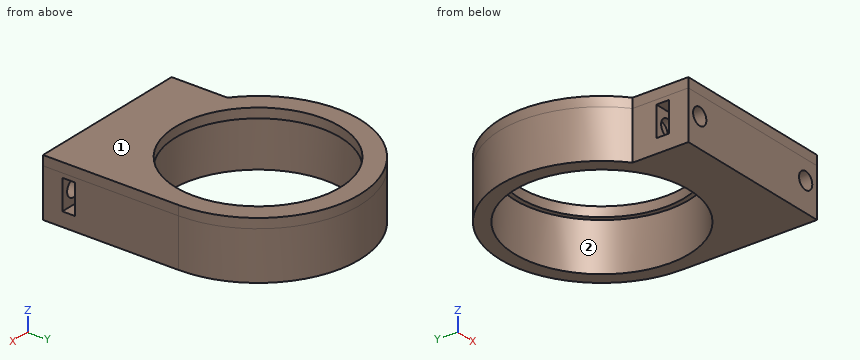
```python
from build123d import *
from build123d.topology import SkipClean

# Parameters (mm, degrees)
CROQUIS1_R              = 18
SALIENTE_EXTRUIR1_DEPTH = 10
CROQUIS2_R              = 17
SALIENTE_EXTRUIR2_DEPTH = 2
CROQUIS7_R              = 1.75
CORTAR_EXTRUIR3_DEPTH   = 8
CORTAR_EXTRUIR4_DEPTH   = 2.6


with BuildPart() as part:
    # Croquis1 → Saliente-Extruir1 (new body)
    with BuildSketch(Plane.XY):
        with BuildLine():
            Line((-13, -28), (21, -28))
            Line((21, -28), (21, 0))
            ThreePointArc((21, 0), (-9.16515139, 18.894443628), (-13, -16.492422502))
            Line((-13, -16.492422502), (-13, -28))
        make_face()
        Circle(CROQUIS1_R, mode=Mode.SUBTRACT)
    extrude(amount=SALIENTE_EXTRUIR1_DEPTH)

    # Croquis2 → Saliente-Extruir2 (add)
    with SkipClean():  # the faces are left unmerged after this step: merging them gives an invalid solid
        with BuildSketch(Plane.XY.offset(10)):
            with BuildLine():
                Line((21, 0), (21, -28))
                Line((21, -28), (-13, -28))
                Line((-13, -28), (-13, -16.492422502))
                ThreePointArc((-13, -16.492422502), (-9.16515139, 18.894443628), (21, 0))
            make_face()
            Circle(CROQUIS2_R, mode=Mode.SUBTRACT)
        extrude(amount=SALIENTE_EXTRUIR2_DEPTH)

    # Croquis7 → Cortar-Extruir3 (cut)
    with SkipClean():  # the faces are left unmerged after this step: merging them gives an invalid solid
        with BuildSketch(Plane.XZ.offset(28)):
            with Locations((-10, 6)):
                Circle(CROQUIS7_R)
            with Locations((18, 6)):
                Circle(CROQUIS7_R)
        extrude(amount=-CORTAR_EXTRUIR3_DEPTH, mode=Mode.SUBTRACT)

    # Croquis8 → Cortar-Extruir4 (cut)
    with SkipClean():  # the faces are left unmerged after this step: merging them gives an invalid solid
        with BuildSketch(Plane(origin=(0, -24, 0), x_dir=(-1, 0, 0), z_dir=(0, -1, 0))):
            with BuildLine():
                Line((-18, -2.9), (-21, -2.9))
                Line((-21, -2.9), (-21, -9.1))
                Line((-21, -9.1), (-18, -9.1))
                ThreePointArc((-18, -9.1), (-14.9, -6), (-18, -2.9))
            make_face()
            with BuildLine():
                Line((10, -2.9), (13, -2.9))
                Line((13, -2.9), (13, -9.1))
                Line((13, -9.1), (10, -9.1))
                ThreePointArc((10, -9.1), (6.9, -6), (10, -2.9))
            make_face()
        extrude(amount=-CORTAR_EXTRUIR4_DEPTH, mode=Mode.SUBTRACT)


solid = part.part
```
Geometry: final body of the model. Coordinates: model frame, mm. Face numbers are marked on the shaded views. A direction names the side the tool comes from. Coordinates: 2 decimals unless noted, no trailing zeros. Order: outer loops, then holes, each group sorted by start corner. A loop starts at its lowest first (then second) coordinate and runs counter-clockwise, first axis right, second up. Notation, with made-up numbers: M 83.25,5.25 L 107.25,5.25 A24 cw 107.25,33.25 Z; hole C -28,-24.5 d11. An arc over 180 degrees is marked long. Answer in a Markdown table with one row per item. Add a question column.
Q1. Line query: L1, parallel to Y at x = 0, z = 10.95; L2, parallel to X at y = 0.5, z = 2; L3, parallel to Z at x = -10, y = -21.1. Output: solid intervals per line, ascending.
Q2. Contact query for flat-ended pins moving along their axis: P1, Ø2, axis at y = 6, z = 1.5, coming from the -X side; P2, Ø1.8, axis at x = -11, z = 4.5, coming from the +Y side; P3, Ø2, axis at x = -10, z = 6, coming from the +Y side. Output: stop coordinate, or through.
Q3. Section query B-B on x = -7.5. Return the cut outline in (y, z), and give its area (3 significant figures).
Q4. Reachability of the marked faces 1 and 2 from +Z, -Z, +X, -X, +Y, -Y: full face, straight path, thin tool, end or side. Return the list, or none.
Q5. Section query C-C on x = 0. Return the cut outline in (y, z), and give its area (3 significant figures).
Q6. Section query A-A on z = 6. Count the separate pieces of the cut face and the enclosed holes in it, and give its area (3 significant figures).
Q7. Section query D-D on y = -10.5. Return the cut outline in (x, z).
Completed:
| question | item | result |
|---|---|---|
| 1 | L1 | y = -28 to -17, 17 to 21 |
| 1 | L2 | x = -20.99 to -17.99, 17.99 to 20.99 |
| 1 | L3 | z = 0 to 4.25, 7.75 to 12 |
| 2 | P1 | stops at x = -20.4 |
| 2 | P2 | stops at y = 18.41 |
| 2 | P3 | stops at y = 18.97 |
| 3 | outline | M -28,0 L -16.36,0 L -16.36,10 L -15.26,10 L -15.26,12 L -28,12 Z; M 15.26,10 L 16.36,10 L 16.36,0 L 19.62,0 L 19.62,12 L 15.26,12 Z; hole M -24,4.17 L -21.4,4.17 L -21.4,7.83 L -24,7.83 Z |
| 3 | area | 174 mm2 |
| 4 | face 1 | +Z, +X, -X, +Y, -Y |
| 4 | face 2 | -Z |
| 5 | outline | M -28,0 L -18,0 L -18,10 L -17,10 L -17,12 L -28,12 Z; M 17,10 L 18,10 L 18,0 L 21,0 L 21,12 L 17,12 Z |
| 5 | area | 160 mm2 |
| 6 | separate pieces | 3 |
| 6 | enclosed holes | 1 |
| 6 | area | 649 mm2 |
| 7 | outline | M -18.19,0 L -14.62,0 L -14.62,10 L -13.37,10 L -13.37,12 L -18.19,12 Z; M 13.37,10 L 14.62,10 L 14.62,0 L 21,0 L 21,12 L 13.37,12 Z |
